Part model, mm, in its own coordinate system. Face numbers are marked on the shaded views. A direction names the side the tool comes from. Give positions to 0.01 mm unless a question says otherwise; leave off trailing zeros. Loops run counter-clockwise (first coordinate to the right, second up) from the corner with the lowest first, then second, coordinate; pieces in that order, holes last. Notation, with made-up numbers: M 88.5,-4.5 L 128.5,-4.5 A29 cw 128.5,18.5 Z; hole C 55.25,-10.5 d1. An arc over 180 degrees is marked long. Answer in a Markdown table with one row per item.
from build123d import *

# Parameters (mm, degrees)
BOSS_EXTRUDE2_DEPTH = 10


with BuildPart() as part:
    # Sketch1 → Boss-Extrude2 (new body)
    with BuildSketch(Plane.XY):
        with BuildLine():
            Line((39.686269666, -5), (49.749371855, -5))
            ThreePointArc((49.749371855, -5), (48.907380037, -10.395584541), (47.481995894, -15.667165215))
            Line((47.481995894, -15.667165215), (38.2888946, -11.574132812))
            ThreePointArc((38.2888946, -11.574132812), (36.541818306, -16.269465723), (34.221528169, -20.709587388))
            Line((34.221528169, -20.709587388), (43.414629464, -24.802619792))
            ThreePointArc((43.414629464, -24.802619792), (40.450849719, -29.389262615), (37.004551483, -33.625335233))
            Line((37.004551483, -33.625335233), (30.271021813, -26.146992913))
            ThreePointArc((30.271021813, -26.146992913), (26.765224254, -29.725793019), (22.839573558, -32.838298977))
            Line((22.839573558, -32.838298977), (29.573103228, -40.316641297))
            ThreePointArc((29.573103228, -40.316641297), (25, -43.301270189), (20.128683944, -45.769379313))
            Line((20.128683944, -45.769379313), (17.019014352, -36.198800401))
            ThreePointArc((17.019014352, -36.198800401), (12.360679775, -38.042260652), (7.508449189, -39.288970345))
            Line((7.508449189, -39.288970345), (10.618118781, -48.859549256))
            ThreePointArc((10.618118781, -48.859549256), (5.226423163, -49.726094768), (-0.227615912, -49.999481907))
            Line((-0.227615912, -49.999481907), (0.824264696, -39.991506445))
            ThreePointArc((0.824264696, -39.991506445), (-4.181138531, -39.780875815), (-9.120954258, -38.946221812))
            Line((-9.120954258, -38.946221812), (-10.172834865, -48.954197275))
            ThreePointArc((-10.172834865, -48.954197275), (-15.450849719, -47.552825815), (-20.544558909, -45.584219849))
            Line((-20.544558909, -45.584219849), (-15.513007814, -36.869317712))
            ThreePointArc((-15.513007814, -36.869317712), (-20, -34.641016151), (-24.173261852, -31.869317712))
            Line((-24.173261852, -31.869317712), (-29.204812947, -40.584219849))
            ThreePointArc((-29.204812947, -40.584219849), (-33.456530318, -37.157241274), (-37.309161029, -33.287032059))
            Line((-37.309161029, -33.287032059), (-29.167940342, -27.372089))
            ThreePointArc((-29.167940342, -27.372089), (-32.360679775, -23.511410092), (-35.045792865, -19.281919056))
            Line((-35.045792865, -19.281919056), (-43.187013552, -25.196862116))
            ThreePointArc((-43.187013552, -25.196862116), (-45.677272882, -20.336832154), (-47.622670264, -15.234214023))
            Line((-47.622670264, -15.234214023), (-37.779471002, -13.141977432))
            ThreePointArc((-37.779471002, -13.141977432), (-39.125904029, -8.316467633), (-39.85858791, -3.360501425))
            Line((-39.85858791, -3.360501425), (-49.701787172, -5.452738016))
            ThreePointArc((-49.701787172, -5.452738016), (-50, 0), (-49.701787172, 5.452738016))
            Line((-49.701787172, 5.452738016), (-39.85858791, 3.360501425))
            ThreePointArc((-39.85858791, 3.360501425), (-39.125904029, 8.316467633), (-37.779471002, 13.141977432))
            Line((-37.779471002, 13.141977432), (-47.622670264, 15.234214023))
            ThreePointArc((-47.622670264, 15.234214023), (-45.677272882, 20.336832154), (-43.187013552, 25.196862116))
            Line((-43.187013552, 25.196862116), (-35.045792865, 19.281919056))
            ThreePointArc((-35.045792865, 19.281919056), (-32.360679775, 23.511410092), (-29.167940342, 27.372089))
            Line((-29.167940342, 27.372089), (-37.309161029, 33.287032059))
            ThreePointArc((-37.309161029, 33.287032059), (-33.456530318, 37.157241274), (-29.204812947, 40.584219849))
            Line((-29.204812947, 40.584219849), (-24.173261852, 31.869317712))
            ThreePointArc((-24.173261852, 31.869317712), (-20, 34.641016151), (-15.513007814, 36.869317712))
            Line((-15.513007814, 36.869317712), (-20.544558909, 45.584219849))
            ThreePointArc((-20.544558909, 45.584219849), (-15.450849719, 47.552825815), (-10.172834865, 48.954197275))
            Line((-10.172834865, 48.954197275), (-9.120954258, 38.946221812))
            ThreePointArc((-9.120954258, 38.946221812), (-4.181138531, 39.780875815), (0.824264696, 39.991506445))
            Line((0.824264696, 39.991506445), (-0.227615912, 49.999481907))
            ThreePointArc((-0.227615912, 49.999481907), (5.226423163, 49.726094768), (10.618118781, 48.859549256))
            Line((10.618118781, 48.859549256), (7.508449189, 39.288970345))
            ThreePointArc((7.508449189, 39.288970345), (12.360679775, 38.042260652), (17.019014352, 36.198800401))
            Line((17.019014352, 36.198800401), (20.128683944, 45.769379313))
            ThreePointArc((20.128683944, 45.769379313), (25, 43.301270189), (29.573103228, 40.316641297))
            Line((29.573103228, 40.316641297), (22.839573558, 32.838298977))
            ThreePointArc((22.839573558, 32.838298977), (26.765224254, 29.725793019), (30.271021813, 26.146992913))
            Line((30.271021813, 26.146992913), (37.004551483, 33.625335233))
            ThreePointArc((37.004551483, 33.625335233), (40.450849719, 29.389262615), (43.414629464, 24.802619792))
            Line((43.414629464, 24.802619792), (34.221528169, 20.709587388))
            ThreePointArc((34.221528169, 20.709587388), (36.541818306, 16.269465723), (38.2888946, 11.574132812))
            Line((38.2888946, 11.574132812), (47.481995894, 15.667165215))
            ThreePointArc((47.481995894, 15.667165215), (48.907380037, 10.395584541), (49.749371855, 5))
            Line((49.749371855, 5), (39.686269666, 5))
            ThreePointArc((39.686269666, 5), (40, 0), (39.686269666, -5))
        make_face()
        with BuildLine():
            Line((-5, 24.494897428), (-5, 28))
            Line((-5, 28), (5, 28))
            Line((5, 28), (5, 24.494897428))
            ThreePointArc((5, 24.494897428), (0, -25), (-5, 24.494897428))
        make_face(mode=Mode.SUBTRACT)
    extrude(amount=BOSS_EXTRUDE2_DEPTH)


solid = part.part
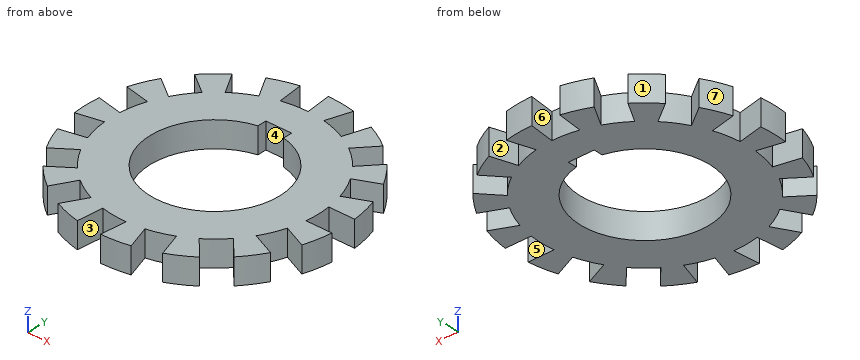
(1) Saw through at C-C (y = 30.5). Write the cut outline in (x, z), plus the area to 3 significant figures.
Recorded:
| item | result |
|---|---|
| outline | M -33.47,0 L 25.88,0 L 25.88,10 L -33.47,10 Z; M 34.19,0 L 39.62,0 L 39.62,10 L 34.19,10 Z |
| area | 648 mm^2 |
(2) Saw through at D-D (x = -27). Write the cut outline in (y, z), plus the area to 3 significant figures.
Recorded:
| item | result |
|---|---|
| outline | M -36.77,0 L 36.77,0 L 36.77,10 L -36.77,10 Z |
| area | 735 mm^2 |
(3) Saw through at A-A (y = 0). Write the cut outline in (x, z), plus the area to 3 significant figures.
Recorded:
| item | result |
|---|---|
| outline | M -50,0 L -25,0 L -25,10 L -50,10 Z; M 25,0 L 40,0 L 40,10 L 25,10 Z |
| area | 400 mm^2 |
(4) Pin check, flat tips, straight feed: pin 1 Ø3 at (y, z) = (26.5, 7) entering from +X; pin 2 Ø1 at (x, z) = (33, 7) entering from -Y; pin 3 Ø3 at (x, z) = (1.5, 2.5) entering from -Y. Stop position of each tip, or through.
Recorded:
| item | result |
|---|---|
| pin 1 | stops at x = 43.3 |
| pin 2 | stops at y = -29.73 |
| pin 3 | stops at y = -50 |
(5) Saw through at B-B (y = -44). Write the cut outline in (x, z), plus the area to 3 significant figures.
Recorded:
| item | result |
|---|---|
| outline | M -19.63,0 L -9.65,0 L -9.65,10 L -19.63,10 Z; M 0.4,0 L 9.04,0 L 9.04,10 L 0.4,10 Z; M 19.55,0 L 23.75,0 L 23.75,10 L 19.55,10 Z |
| area | 228 mm^2 |
(6) Pull direction X, two halves, no side cores. Call the marked faces 5, 6 and 7: +X half, -X half, draft (parallel to the pull), parting line (faces both ways), or undercut.
Recorded:
| item | result |
|---|---|
| face 5 | draft |
| face 6 | undercut |
| face 7 | -X half |
(7) Which spindle directions (+Z, -Z, +X, -X, +Y, -Y) get a long thin tool onto all of the face, cutting with end or side? Do the marked faces 1, 2, 3 and 4. Say none if no direction does.
Recorded:
| item | result |
|---|---|
| face 1 | +Z, -Z, -X, +Y |
| face 2 | +Z, -Z, +Y |
| face 3 | +Z, -Z, -Y |
| face 4 | +Z, -Z |
(8) Drill centre lines: line 1 along Y through (x, z) = (-36.5, 6); line 2 along Y through (x, z) = (43, 1); line 3 along X through (y, z) = (-15.5, 7.25). Where is each one in solid material? Low to high.
Recorded:
| item | result |
|---|---|
| line 1 | y = -34.17 to -32.7, -20.34 to 20.34, 32.7 to 34.17 |
| line 2 | y = -25.51 to -24.62, -13.67 to -5, 5 to 13.67, 24.62 to 25.51 |
| line 3 | x = -47.54 to -19.62, 19.62 to 36.87, 47.11 to 47.54 |
